Geometry check sheet. Reference: drawing and pictorial views, mm from the part's lowest x, y, z. A direction names the side the tool comes from. Coordinates: 2 decimals unless noted, no trailing zeros. Write each loop counter-clockwise with the first axis right and the second up, starting at its lowest first coordinate (ties: lowest second). Pieces come first, ordered by that corner, then holes.
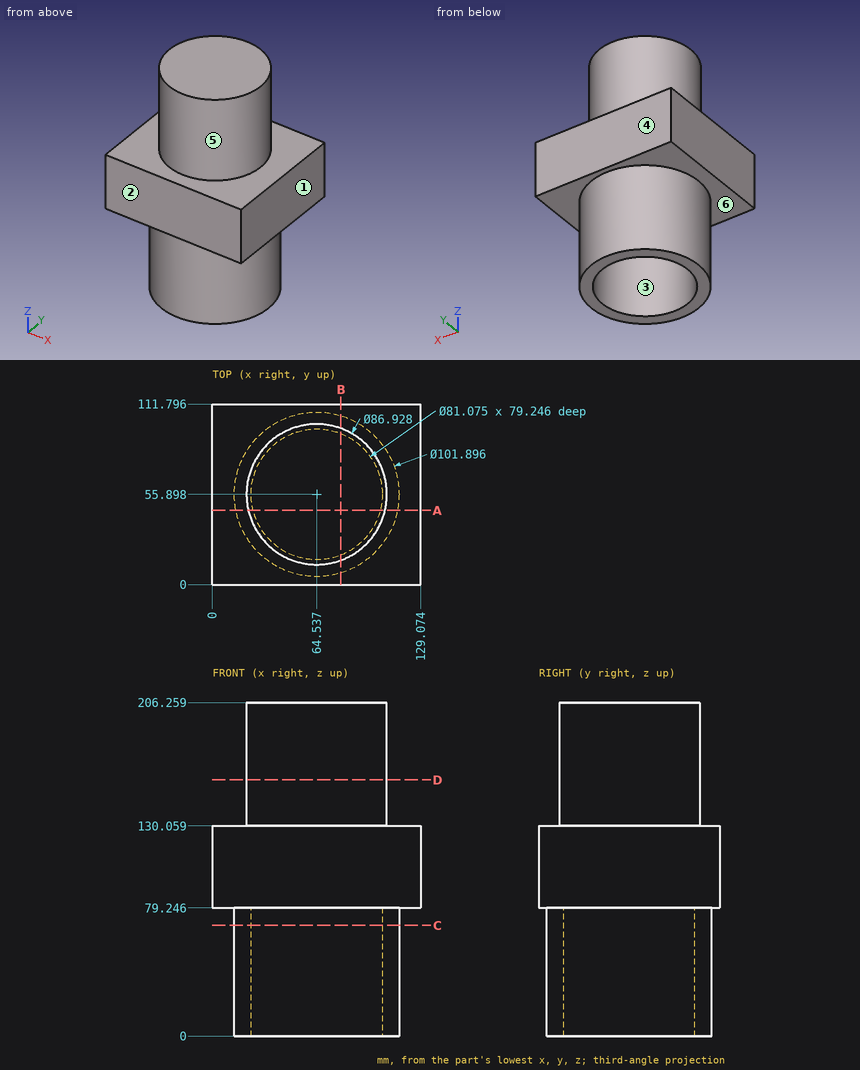
1. Sectioned sample at B-B, the plane x = 79.5. Record the boundary of the cut face in (y, z) (1 decimal).
2. Gauge pin test, flat ends, axial feed: P1, Ø2, axis at x = 88.5, y = 62.5, coming from the -Z side; P2, Ø2, axis at x = 36.5, z = 151.5, coming from the -Y side (1 decimal); P3, Ø8, axis at y = 61.5, z = 40, coming from the -X side. Record the tip position at first contact, or that the pin passes through.
3. Material ranges on L1, parallel to Z at x = 114.5, y = 27 (1 decimal); L2, parallel to Z at x = 77, y = 31.5 (1 decimal); L3, parallel to Y at x = 49.5, z = 52.5 (1 decimal), recorded low to high.
4. Draft check along Y on the marked faces 1, 2 and 3. Enter one of: pulls with the +Y half, pulls with the -Y half, needs draft (parallel to the pull), parting line crosses it, or undercut.
5. Sectioned sample at C-C, the plane z = 68.5. Record the boundary of the cut face in (x, y) (1 decimal), and give its area (3 significant figures).
6. Sectioned sample at A-A, the plane y = 46. Record the boundary of the cut face in (x, z) (1 decimal), and give its area (3 significant figures).
7. Sectioned sample at D-D, the plane z = 158.5. Record the boundary of the cut face in (x, y) (1 decimal).
8. Tool access check on the marked faces 4, 5 and 6. Record the directions out of +Z, -Z, +X, -X, +Y, -Y that give a thin tool (end or side, any length) a straight path to the whole face; none if there is none.
Outcome:
1. outline: (0, 79.2) - (7.2, 79.2) - (7.2, 0) - (18.2, 0) - (18.2, 79.2) - (93.6, 79.2) - (93.6, 0) - (104.6, 0) - (104.6, 79.2) - (111.8, 79.2) - (111.8, 130.1) - (96.7, 130.1) - (96.7, 206.3) - (15.1, 206.3) - (15.1, 130.1) - (0, 130.1) - close
2. P1: stops at z = 79.25
2. P2: stops at y = 21.9
2. P3: stops at x = 13.61
3. L1: z = 79.2 to 130.1
3. L2: z = 79.2 to 206.3
3. L3: y = 7.2 to 18.3, 93.5 to 104.6
4. face 1: needs draft
4. face 2: pulls with the -Y half
4. face 3: undercut
5. outline: circle Ø101.9 at (64.5, 55.9); hole circle Ø81.1 at (64.5, 55.9)
5. area: 2,990 mm2
6. outline: (0, 79.2) - (14.6, 79.2) - (14.6, 0) - (25.2, 0) - (25.2, 79.2) - (103.8, 79.2) - (103.8, 0) - (114.5, 0) - (114.5, 79.2) - (129.1, 79.2) - (129.1, 130.1) - (106.9, 130.1) - (106.9, 206.3) - (22.2, 206.3) - (22.2, 130.1) - (0, 130.1) - close
6. area: 14,700 mm2
7. outline: circle Ø86.9 at (64.5, 55.9)
8. face 4: +Z, -Z, +X, -X, +Y
8. face 5: +Z
8. face 6: -Z
